Model file for the job. Use its own axes, mm. Face numbers are marked on the shaded views. Coordinates: 2 decimals unless noted, no trailing zeros. Order: outer loops, then holes, each group sorted by start corner. A loop starts at its lowest first (then second) coordinate and runs counter-clockwise, first axis right, second up. Notation, with made-up numbers: (-17.5, 27.25) -> (29.5, 27.25) arc R22 ccw to (29.5, 34.25) -> close; hole circle Ø4 at (-35.75, 66.25). An arc over 180 degrees is marked (long way). Use CSV: the item, a comma, the result in double quotes. Start each with the question number.
(1) Cut at B-B on x = -59. Write the cut outline in (y, z), plus the area to 3 significant figures.
(2) Probe L1, parallel to Z at x = -132, y = 17.25; L2, parallel to Z at x = -134.5, y = 9; L3, parallel to Z at x = -68, y = 22.75. List the from-to ranges inside material, lowest first.
(3) Cut at D-D on y = 11.25. Write the cut outline in (x, z), plus the area to 3 significant figures.
(4) Cut at C-C on x = -128.5. Write the cut outline in (y, z).
(5) Pull direction X, two halves, no side cores. Call the marked faces 1, 2 and 3: pulls with the +X half, pulls with the -X half, needs draft (parallel to the pull), parting line crosses it, or undercut.
(6) Cut at A-A on z = -48. Write the cut outline in (x, y), plus the area to 3 significant figures.
(7) Pin check, flat tips, straight feed: pin 1 Ø10 at (y, z) = (16.5, -6) entering from +X; pin 2 Ø4 at (x, y) = (-123.5, 9.5) entering from +Z; pin 3 Ø10 at (x, y) = (-95.5, 16) entering from +Z. Stop position of each tip, or through.
```python
from build123d import *

# Parameters (mm, degrees)
SZKIC1_R                    = 8
DODANIE_WYCI_GNI_CIE1_DEPTH = 25
SZKIC2_R                    = 6
WYTNIJ_WYCI_GNI_CIE1_DEPTH  = 25
SZKIC3_R                    = 8
WYTNIJ_WYCI_GNI_CIE2_DEPTH  = 2000


with BuildPart() as part:
    # Szkic1 → Dodanie-wyciągnięcie1 (new body)
    with BuildSketch(Plane(origin=(0, 0, 0), x_dir=(1, 0, 0), z_dir=(0, 1, 0))):
        with BuildLine():
            Line((-145.921678768, -1.827473833), (-139.75350446, 83.413416114))
            ThreePointArc((-139.75350446, 83.413416114), (-95.818169931, 143.778859358), (-22.261154385, 130.985664988))
            Line((-22.261154385, 130.985664988), (-13.598892288, 123.247376031))
            ThreePointArc((-13.598892288, 123.247376031), (-12.564771829, 104.891706747), (-30.920441114, 103.857586288))
            Line((-30.920441114, 103.857586288), (-39.58270321, 111.595875245))
            ThreePointArc((-39.58270321, 111.595875245), (-86.060369899, 119.679371012), (-113.821309069, 81.536918796))
            Line((-113.821309069, 81.536918796), (-119.989483377, -3.703971151))
            ThreePointArc((-119.989483377, -3.703971151), (-133.893829731, -15.731820187), (-145.921678768, -1.827473833))
        make_face()
        with Locations((-132.955581072, -2.765722492)):
            Circle(SZKIC1_R, mode=Mode.SUBTRACT)
        with Locations((-22.259666701, 113.552481159)):
            Circle(SZKIC1_R, mode=Mode.SUBTRACT)
    extrude(amount=DODANIE_WYCI_GNI_CIE1_DEPTH)

    # Szkic2 → Wytnij-wyciągnięcie1 (cut)
    with BuildSketch(Plane(origin=(0, 25, 0), x_dir=(1, 0, 0), z_dir=(0, 1, 0))):
        with Locations((-56.034895704, 134.982224644)):
            Circle(SZKIC2_R)
    extrude(amount=-WYTNIJ_WYCI_GNI_CIE1_DEPTH, mode=Mode.SUBTRACT)

    # Szkic3 → Wytnij-wyciągnięcie2 (cut)
    with BuildSketch(Plane(origin=(0, 25, 0), x_dir=(1, 0, 0), z_dir=(0, 1, 0))):
        with Locations((-129.654921114, 42.234277508)):
            Circle(SZKIC3_R)
    extrude(amount=-WYTNIJ_WYCI_GNI_CIE2_DEPTH, mode=Mode.SUBTRACT)


solid = part.part
```
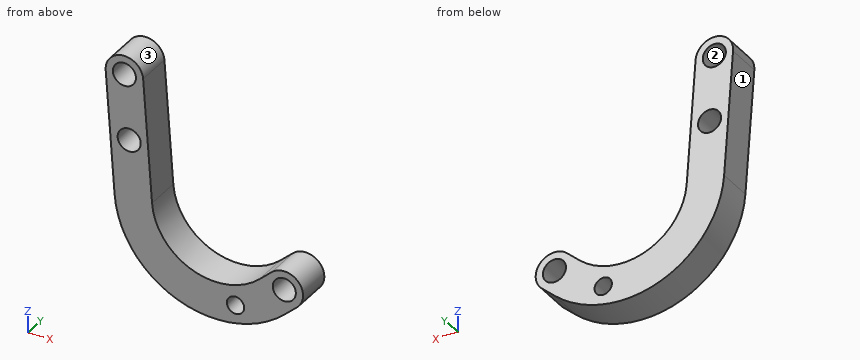
Outcome:
1,outline,"(0, -148.18) -> (25, -148.18) -> (25, -140.2) -> (0, -140.2) -> close; (0, -129.77) -> (25, -129.77) -> (25, -121.73) -> (0, -121.73) -> close"
1,area,"400 mm2"
2,L1,"-110.85 to -49.88, -34.59 to -5.18, 10.71 to 15.73"
2,L2,"-105.49 to -48.6, -35.87 to -5.08, 10.62 to 15.67"
2,L3,"-148.93 to -122.92"
3,outline,"(-145.92, 1.83) -> (-139.75, -83.41) arc R70.63 ccw to (-22.26, -130.99) -> (-13.6, -123.25) arc R13 ccw to (-30.92, -103.86) -> (-39.58, -111.6) arc R44.63 cw to (-113.82, -81.54) -> (-119.99, 3.7) arc R13 ccw to start; hole circle Ø16 at (-132.96, 2.77); hole circle Ø16 at (-129.65, -42.23); hole circle Ø12 at (-56.03, -134.98); hole circle Ø16 at (-22.26, -113.55)"
3,area,"5,680 mm2"
4,outline,"(0, -116.85) -> (25, -116.85) -> (25, -50.15) -> (0, -50.15) -> close; (0, -34.32) -> (25, -34.32) -> (25, -3.88) -> (0, -3.88) -> close; (0, 9.41) -> (25, 9.41) -> (25, 14.98) -> (0, 14.98) -> close"
5,face 1,"pulls with the -X half"
5,face 2,"undercut"
5,face 3,"parting line crosses it"
6,outline,"(-142.32, 0) -> (-135.2, 0) -> (-135.2, 25) -> (-142.32, 25) -> close; (-124.11, 0) -> (-116.25, 0) -> (-116.25, 25) -> (-124.11, 25) -> close"
6,area,"374 mm2"
7,pin 1,"x = -118.93"
7,pin 2,"z = 13.42"
7,pin 3,"z = -110.23"
